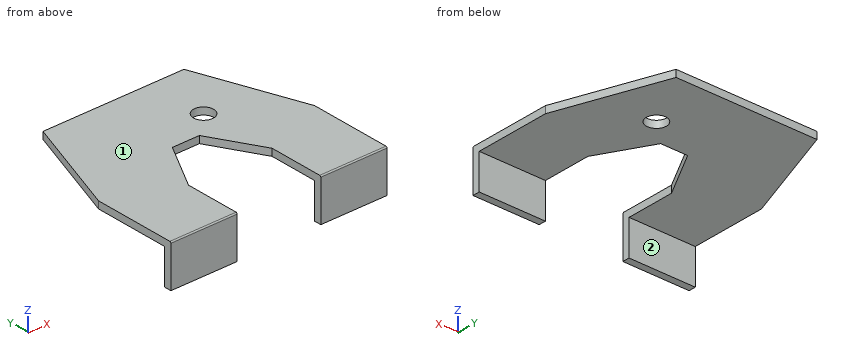
```python
from build123d import *

# Parameters (mm, degrees)
CROQUIS1_R              = 4.271780476
SALIENTE_EXTRUIR1_DEPTH = 3
CROQUIS2_W              = 28.196158727
CROQUIS2_H              = 3
SALIENTE_EXTRUIR2_DEPTH = 15
REDONDEO1_R             = 0.5


with BuildPart() as part:
    # Croquis1 → Saliente-Extruir1 (new body)
    with BuildSketch(Plane.XY):
        Polygon((-46, -40), (-46, -5), (-30, 40), (30, 40), (46, -5), (46, -40), (17.803841273, -40), (17.803841273, -16.484284277), (5.75, 5), (-5.75, 5), (-17.803841273, -16.484284277), (-17.803841273, -40), align=None)
        with Locations((16, 14.6)):
            Circle(CROQUIS1_R, mode=Mode.SUBTRACT)
    extrude(amount=SALIENTE_EXTRUIR1_DEPTH)

    # Croquis2 → Saliente-Extruir2 (add)
    with BuildSketch(Plane(origin=(0, 0, 0), x_dir=(-1, 0, 0), z_dir=(0, 0, -1))):
        with Locations((-31.901920637, -38.5)):
            Rectangle(CROQUIS2_W, CROQUIS2_H)
        with Locations((31.901920637, -38.5)):
            Rectangle(CROQUIS2_W, CROQUIS2_H)
    extrude(amount=SALIENTE_EXTRUIR2_DEPTH)

    # Redondeo1
    redondeo1_edges = [part.edges().sort_by_distance(p)[0] for p in [
        (-31.901920636, -40, 3),
        (31.901920636, -40, 3),
    ]]
    fillet(redondeo1_edges, radius=REDONDEO1_R)


solid = part.part
```
The listing builds one solid part. Answer for the finished solid, in the listing's coordinates (mm). Face numbers are marked on the shaded views. A direction names the side the tool comes from. Round coordinates to 2 decimals unless told otherwise and drop trailing zeros. Write each loop counter-clockwise with the first axis right and the second up, starting at its lowest first coordinate (ties: lowest second). Pieces come first, ordered by that corner, then holes. Notation, with made-up numbers: (87, 3.25) -> (103, 3.25) arc R29 ccw to (103, 32.25) -> close; hole circle Ø11 at (9.5, 73). An arc over 180 degrees is marked (long way). Use CSV: the item, a comma, the result in double quotes. Start each with the question number.
(1) Section C-C on x = -3 is taken. Give the vertices of the cut face in (y, z).
(2) Consider L1, parallel to Z at x = 41.5, y = -7.5; L2, parallel to Y at x = 16, z = 2.2; L3, parallel to Y at x = -25.5, z = -7.25. Determine where each line is inside the solid, lowest interval first. Write a range as from..to.
(3) Section B-B on x = 16 is taken. Give the vertices of the cut face in (y, z), then the cut area to 3 significant figures.
(4) Each of these flat-tipped pins is pushed along its axis until it touches: pin 1 (0.9 mm diameter, centred on x = -1.5, z = 2, fed in from -Y); pin 2 (4.5 mm diameter, centred on x = 32.5, z = -5, fed in from +Y); pin 3 (4 mm diameter, centred on x = -26, y = 31, fed in from -Z). Where does it stop, or does it pass through?
(5) Which of the six approach directions +Z, -Z, +X, -X, +Y, -Y give full straight-line access (tool end or side, diameter ignored) to the marked faces 1 and 2?
(6) Section D-D on y = 6 is taken. Give the vertices of the cut face in (x, z), then the cut area to 3 significant figures.
(7) Section A-A on z = -6.5 is taken. Give the vertices of the cut face in (x, y), then the cut area to 3 significant figures.
A:
1,outline,"(5, 0) -> (40, 0) -> (40, 3) -> (5, 3) -> close"
2,L1,"z = 0..3"
2,L2,"y = -13.27..10.33, 18.87..40"
2,L3,"y = -40..-37"
3,outline,"(-13.27, 0) -> (10.33, 0) -> (10.33, 3) -> (-13.27, 3) -> close; (18.87, 0) -> (40, 0) -> (40, 3) -> (18.87, 3) -> close"
3,area,"134 mm²"
4,pin 1,"stops at y = 5"
4,pin 2,"stops at y = -37"
4,pin 3,"stops at z = 0"
5,face 1,"+Z, +X, -X, +Y, -Y"
5,face 2,"-Z, +X, -X, +Y"
6,outline,"(-42.09, 0) -> (42.09, 0) -> (42.09, 3) -> (-42.09, 3) -> close"
6,area,"253 mm²"
7,outline,"(-46, -40) -> (-17.8, -40) -> (-17.8, -37) -> (-46, -37) -> close; (17.8, -40) -> (46, -40) -> (46, -37) -> (17.8, -37) -> close"
7,area,"169 mm²"
